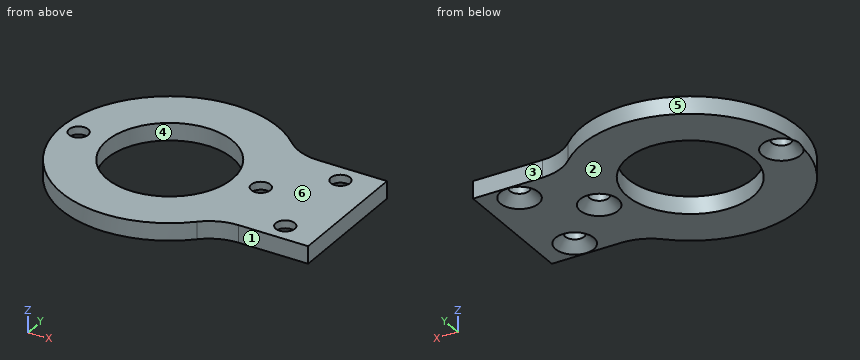
Autodesk Inventor part; units mm, degrees
ref_plane "YZ Plane" through (0, 0, 0) normal (1, 0, 0) x (0, 1, 0)
ref_plane "XZ Plane" through (0, 0, 0) normal (0, 1, 0) x (-1, 0, 0)
ref_plane "XY Plane" through (0, 0, 0) normal (0, 0, 1) x (1, 0, 0)
sketch "Skizze1" plane through (0, 0, 0) normal (0, 0, 1) x (1, 0, 0)
  line L0 (0, 0) -> (20.5, 0) construction
  circle A0 centre (0, 0) radius 7.25
  arc A1 (8.6207, 9.0517) -> (12.5, 7.5) centre (12.5, 13.125) ccw
  arc A2 (12.5, -7.5) -> (8.6207, -9.0517) centre (12.5, -13.125) ccw
  line L1 (12.5, 7.5) -> (20.5, 7.5)
  line L2 (20.5, 7.5) -> (20.5, -7.5)
  line L3 (20.5, -7.5) -> (12.5, -7.5)
  line L4 (12.5, -7.5) -> (12.5, 7.5) construction
  circle A3 centre (0, 0) radius 10.5 construction
  line L5 (0, 0) -> (-10.5, 0) construction
  line L6 (16.5, 5.25) -> (16.5, -5.25) construction
  line L7 (16.5, 7.5) -> (16.5, -7.5) construction
  circle A4 centre (0, 0) radius 12.5
  point P0 (12.5, 0)
  point P1 (10.5, 0)
  point P2 (16.5, 0)
  dimension "d105" = 14.5
  dimension "d106" = 15
  dimension "LowerArm_ShaftFixation_Width" = 8
  dimension "d127" = 21
  dimension "d130" = 360
  dimension "d132" = 10.5
  dimension "d150" = 25
extrude "Grundprofil" add sketch "Skizze1" along normal blind 2
hole "Hole10" at (10.5, 0, 0) at (-10.5, 0, 0) direction (0, 0, 1) diameter 2.2 depth 12 tip angle 118 countersink diameter 4.4 countersink angle 90
hole "Hole11" at (16.5, 5.25, 0) at (16.5, -5.25, 0) direction (0, 0, 1) diameter 2.2 depth 3 tip angle 118 countersink diameter 4.4 countersink angle 90
properties part number "Lower_Arm_v4" material "Aluminum 6061"
Input: part model. Units: mm. Frame: model coordinates. Face numbers are marked on the shaded views. A direction names the side the tool comes from. Give positions to 0.01 mm unless a question says otherwise; leave off trailing zeros. Loops run counter-clockwise (first coordinate to the right, second up) from the corner with the lowest first, then second, coordinate; pieces in that order, holes last. Notation, with made-up numbers: M 77,30 L 119,30 A15 cw 119,41 Z; hole C -2,2.5 d6. An arc over 180 degrees is marked long. Answer as CSV lines item,"result". Start each with the question number.
1. Pin query (flat end, axial travel): P1, Ø1, axis at x = 4, z = 0.5, coming from the +Y side; P2, Ø1, axis at x = 15.5, z = 1.5, coming from the -Y side; P3, Ø1, axis at x = 18.5, z = 0.5, coming from the +Y side. Return the tip coordinate at first contact, or that it passes through.
2. Section D-D on y = 0. Return loops of the section in (x, z), plus the area to 3 significant figures.
3. Section A-A on x = 0. Return loops of the section in (y, z), plus the area to 3 significant figures.
4. Line query: L1, parallel to Y at x = 16.5, z = 1.35; L2, parallel to Y at x = 0, z = 0.85; L3, parallel to X at y = -6.5, z = 0.15. Output: solid intervals per line, ascending.
5. Section B-B on x = 16.5. Return loops of the section in (y, z).
6. Reachability of the marked faces 1, 2 and 3 from +Z, -Z, +X, -X, +Y, -Y: full face, straight path, thin tool, end or side. Return the list, or none.
7. Section C-C on z = 1.45. Return loops of the section in (x, y), plus the area to 3 significant figures.
8. Pull-direction query (Y, two-part tool) for the marked faces 4, 5 and 6; classes: released by +Y, released by -Y, zero draft, split by the parting line, or undercut.
Computed values:
1,P1,"stops at y = 12"
1,P2,"stops at y = -7.5"
1,P3,"stops at y = 7.5"
2,outline,"M -12.5,0.2 L -11.6,1.1 L -11.6,2 L -12.5,2 Z; M -9.4,1.1 L -8.3,0 L -7.25,0 L -7.25,2 L -9.4,2 Z; M 7.25,0 L 8.3,0 L 9.4,1.1 L 9.4,2 L 7.25,2 Z; M 11.6,1.1 L 12.7,0 L 20.5,0 L 20.5,2 L 11.6,2 Z"
2,area,"25.8 mm²"
3,outline,"M -12.5,0 L -7.25,0 L -7.25,2 L -12.5,2 Z; M 7.25,0 L 12.5,0 L 12.5,2 L 7.25,2 Z"
3,area,"21.0 mm²"
4,L1,"y = -7.5 to -6.35, -4.15 to 4.15, 6.35 to 7.5"
4,L2,"y = -12.5 to -7.25, 7.25 to 12.5"
4,L3,"x = -10.68 to -3.21, 3.21 to 14.88, 18.12 to 20.5"
5,outline,"M -7.5,0 L -7.45,0 L -6.35,1.1 L -6.35,2 L -7.5,2 Z; M -4.15,1.1 L -3.05,0 L 3.05,0 L 4.15,1.1 L 4.15,2 L -4.15,2 Z; M 6.35,1.1 L 7.45,0 L 7.5,0 L 7.5,2 L 6.35,2 Z"
6,face 1,"+Z, -Z, +X, -Y"
6,face 2,"-Z, +X, -X, +Y, -Y"
6,face 3,"+Z, -Z, +X, +Y"
7,outline,"M 8.62,-9.05 A5.63 cw 12.5,-7.5 L 20.5,-7.5 L 20.5,7.5 L 12.5,7.5 A5.62 cw 8.62,9.05 A12.5 ccw long Z; hole C -10.5,0 d2.2; hole C 0,0 d14.5; hole C 10.5,0 d2.2; hole C 16.5,-5.25 d2.2; hole C 16.5,5.25 d2.2"
7,area,"444 mm²"
8,face 4,"undercut"
8,face 5,"split by the parting line"
8,face 6,"zero draft"
